Geometry check sheet. Reference: the model listing, model coordinates, mm. Face numbers are marked on the shaded views. A direction names the side the tool comes from. Round coordinates to 2 decimals unless told otherwise and drop trailing zeros. Write each loop counter-clockwise with the first axis right and the second up, starting at its lowest first coordinate (ties: lowest second). Pieces come first, ordered by that corner, then holes. Notation, with made-up numbers: (38.5, 23.5) -> (89.5, 23.5) arc R18 ccw to (89.5, 48.5) -> close; hole circle Ø7 at (-2, -12). An arc over 180 degrees is marked (long way). One line per question, with ' | ' between items.
```python
from build123d import *

# Parameters (mm, degrees)
BOSS_EXTRUDE1_DEPTH = 25.654
FILLET1_R           = 25.4
FILLET2_R           = 2.54


with BuildPart() as part:
    # Sketch1 → Boss-Extrude1 (new body)
    with BuildSketch(Plane(origin=(0, 0, 0), x_dir=(0, 0, -1), z_dir=(1, 0, 0))):
        Polygon((-4.9845, -12.7), (-2.9845, -12.7), (-2.9845, 0), (2.9845, 0), (2.9845, -25.4), (4.9845, -25.4), (4.9845, 3.175), (-4.9845, 3.175), align=None)
    extrude(amount=BOSS_EXTRUDE1_DEPTH)

    # Fillet1
    # the kernel refuses this fillet: 25.4 mm, written as the material it takes off along each edge
    with BuildSketch(Plane(origin=(-24.69817807, -12.7, 4.9845), x_dir=(0, 0, -1), z_dir=(1, 0, 0))) as fillet1_piece_1:
        with BuildLine():
            CenterArc((25.4, 9.879271228), FILLET1_R, 180, 22.889037196)
            Line((0, 9.879271228), (-0.508, 9.879271228))
            Line((-0.508, 9.879271228), (-0.508, 0))
            Line((-0.508, 0), (0, -0.508))
            ThreePointArc((0, -0.508), (1, -0.508), (1.532, -0.197585425))
            Line((1.532, -0.197585425), (2, 0))
        make_face()
    extrude(amount=75.050356141, mode=Mode.SUBTRACT)
    with BuildSketch(Plane(origin=(-24.69817807, -25.4, -4.9845), x_dir=(0, 0, 1), z_dir=(1, 0, 0))) as fillet1_piece_2:
        with BuildLine():
            CenterArc((25.4, -9.879271228), FILLET1_R, 157.110962804, 22.889037196)
            Line((0, -9.879271228), (-0.508, -9.879271228))
            Line((-0.508, -9.879271228), (-0.508, 0))
            Line((-0.508, 0), (0, 0.508))
            ThreePointArc((0, 0.508), (1, 0.508), (1.532, 0.197585425))
            Line((1.532, 0.197585425), (2, 0))
        make_face()
    extrude(amount=75.050356141, mode=Mode.SUBTRACT)

    # Fillet2
    fillet2_edges = [part.edges().sort_by_distance(p)[0] for p in [
        (12.827, 3.175, 4.9845),
        (12.827, 3.175, -4.9845),
    ]]
    fillet(fillet2_edges, radius=FILLET2_R)


solid = part.part
```
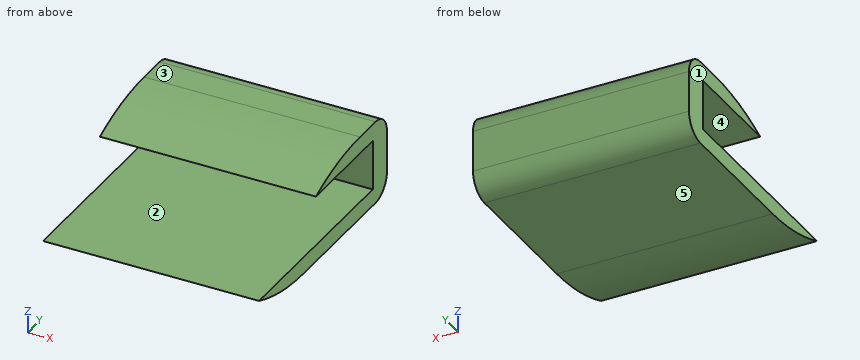
(1) Go/stop test with flat-tipped pins: pin 1 (1.5 mm diameter, centred on x = 7, z = 0, fed in from -Y); pin 2 (1.5 mm diameter, centred on x = 8, y = -17.5, fed in from +Z); pin 3 (4 mm diameter, centred on x = 4, y = -13, fed in from +Z). Record where each tip stops, or that it passes through.
Resolved:
pin 1: stops at y = 0 | pin 2: stops at z = -2.98 | pin 3: stops at z = 3.63
(2) Draft check along Z on the marked faces 1, 2 and 3. Enter one of: +Z half, -Z half, draft (parallel to the pull), parting line (faces both ways), or undercut.
Resolved:
face 1: draft | face 2: undercut | face 3: +Z half
(3) Sectioned sample at D-D on z = 4. Record the cut outline in (x, y), then the cut area to 3 significant figures.
Resolved:
outline: (0, -9.82) -> (25.65, -9.82) -> (25.65, 2.64) -> (0, 2.64) -> close | area: 320 mm2
(4) Material ranges on line 1 (Y direction, x = 21.5, z = 1.75) (3 decimals); line 2 (Z direction, x = 16.5, y = -11.25); line 3 (Z direction, x = 22.5, y = -10), recorded low to high.
Resolved:
line 1: y = 0 to 3.175 | line 2: z = -4.98 to -2.98, 2.98 to 3.55 | line 3: z = -4.98 to -2.98, 2.98 to 3.95
(5) Sectioned sample at A-A on y = -5. Record the cut outline in (x, z).
Resolved:
outline: (0, -4.98) -> (25.65, -4.98) -> (25.65, -2.98) -> (0, -2.98) -> close; (0, 2.98) -> (25.65, 2.98) -> (25.65, 4.89) -> (0, 4.89) -> close
(6) Sectioned sample at B-B on x = 10.25. Record the cut outline in (y, z) (1 decimal).
Resolved:
outline: (-25.4, -3) arc R25.4 ccw to (-15.5, -5) -> (0.6, -5) arc R2.5 ccw to (3.2, -2.4) -> (3.2, 2.4) arc R2.5 ccw to (0.6, 5) -> (-2.8, 5) arc R25.4 ccw to (-12.7, 3) -> (0, 3) -> (0, -3) -> close
(7) Sectioned sample at C-C on y = -14.25. Record the cut outline in (x, z), then the cut area to 3 significant figures.
Resolved:
outline: (0, -4.98) -> (25.65, -4.98) -> (25.65, -2.98) -> (0, -2.98) -> close | area: 51.3 mm2
(8) Access from +Z, -Z, +X, -X, +Y, -Y to the whole of each face (thin tool, end or side, straight path). Record for the marked faces 4 and 5.
Resolved:
face 4: +X, -X, -Y | face 5: -Z, +X, -X, +Y, -Y
